Source: CAD feature listing. Evaluate the final solid. Frame: model axes, mm. A direction names the side the tool comes from. Coordinates: 2 decimals unless noted, no trailing zeros. Order: outer loops, then holes, each group sorted by start corner. A loop starts at its lowest first (then second) coordinate and runs counter-clockwise, first axis right, second up.
```python
from build123d import *

# Parameters (mm, degrees)
F0_R     = 1.5875
F0_W     = 8.89
F0_H     = 11.43
F0_W_2   = 11.43
F0_H_2   = 9.525
F1_DEPTH = 1.6
F0_H_3   = 1.905
F2_DEPTH = 10.9
F0_H_4   = 6.35
F3_DEPTH = 10.75


with BuildPart() as f1:
    # F0 (on Top) → F1 (new body)
    with BuildSketch(Plane.XY):
        Polygon((23.495, 0), (26.67, 0), (26.67, 66.04), (24.13, 66.04), (21.59, 68.58), (-11.176, 68.58), (-13.716, 66.04), (-25.146, 66.04), (-26.67, 64.516), (-26.67, 0), (-17.145, 0), (-17.145, 9.525), (-5.715, 9.525), (-5.715, 0), (14.605, 0), (14.605, 11.43), (23.495, 11.43), align=None)
        with Locations((-24.13, 15.24)):
            Circle(F0_R, mode=Mode.SUBTRACT)
        with Locations((24.13, 13.97)):
            Circle(F0_R, mode=Mode.SUBTRACT)
        with Locations((-8.89, 66.04)):
            Circle(F0_R, mode=Mode.SUBTRACT)
        with Locations((19.05, 66.04)):
            Circle(F0_R, mode=Mode.SUBTRACT)
        with Locations((19.05, 5.715)):
            Rectangle(F0_W, F0_H)
        with Locations((-11.43, 4.7625)):
            Rectangle(F0_W_2, F0_H_2)
    extrude(amount=-F1_DEPTH)

    # F0 (on Top) → F2 (join)
    with BuildSketch(Plane.XY):
        with Locations((19.05, 5.715)):
            Rectangle(F0_W, F0_H)
        with Locations((19.05, -0.9525)):
            Rectangle(F0_W, F0_H_3)
    extrude(amount=F2_DEPTH)

    # F0 (on Top) → F3 (join)
    with BuildSketch(Plane.XY):
        with Locations((-11.43, 4.7625)):
            Rectangle(F0_W_2, F0_H_2)
        with Locations((-11.43, -3.175)):
            Rectangle(F0_W_2, F0_H_4)
    extrude(amount=F3_DEPTH)


solid = f1.part
```
Q1. Set-up query: faces 4 (the flat face through (14.605, 5, 5)), 5 (the flat face through (-12, -3, 0)), 6 (the flat face through (-19, 66.04, -1)), 7 (the flat face through (19, -1.905, 5)), 8 (the flat face through (23.495, 5, 5)). Return all of +Z, -Z, +X, -X, +Y, -Y with unobstructed straight access to the full face (end or side cutting, diameter ignored); none if empty.
Solutions:
face 4: +Z, +Y, -Y
face 5: -Z, +X, -X, -Y
face 6: +Z, -Z, -X, +Y
face 7: +Z, -Z, +X, -Y
face 8: +Z, +X, +Y, -Y
Q2. Pull-direction query (Y, two-part tool) for faces 1 (the cylindrical face through (-9.097, 67.614, -0.789)), 2 (the flat face through (19, 5, 10.9)), 3 (the flat face through (19, 11.43, 5)); classes: pulls with the +Y half, pulls with the -Y half, needs draft (parallel to the pull), parting line crosses it, or undercut.
Solutions:
face 1: undercut
face 2: needs draft
face 3: pulls with the +Y half
Q3. Material intervals for line 1 along X through (y, z) = (1, 9) (3 decimals); line 2 along Y through (x, z) = (-24.13, -1); line 3 along Y through (x, z) = (-8.89, -0.9), sorted ascending.
Solutions:
line 1: x = -17.145 to -5.715, 14.605 to 23.495
line 2: y = 0 to 13.65, 16.83 to 66.04
line 3: y = 0 to 64.45, 67.63 to 68.58
Q4. Section query A-A on x = -24.13. Output: boundary loops of the cut face in (y, z).
Solutions:
outline: (0, -1.6) - (13.65, -1.6) - (13.65, 0) - (0, 0) - close; (16.83, -1.6) - (66.04, -1.6) - (66.04, 0) - (16.83, 0) - close
Q5. Pin query (flat end, axial travel): P1, Ø1.9, axis at x = 24.13, y = 13.97, coming from the -Z side; P2, Ø2.5, axis at x = 18.5, z = 6, coming from the +Y side; P3, Ø0.5, axis at x = -13, z = -1, coming from the -Y side; P4, Ø4, axis at y = 2, z = 8.5, coming from the -X side (3 decimals). Return the tip coordinate at first contact, or that it passes through.
Solutions:
P1: passes through
P2: stops at y = 11.43
P3: stops at y = 0
P4: stops at x = -17.145
Q6. Section query C-C on y = 7.5. Output: boundary loops of the cut face in (x, z) (3 decimals).
Solutions:
outline: (-26.67, -1.6) - (26.67, -1.6) - (26.67, 0) - (23.495, 0) - (23.495, 10.9) - (14.605, 10.9) - (14.605, 0) - (-5.715, 0) - (-5.715, 10.75) - (-17.145, 10.75) - (-17.145, 0) - (-26.67, 0) - close
Q7. Section query B-B on z = 6. Output: boundary loops of the cut face in (x, y) (3 decimals), plus the area to 3 significant figures.
Solutions:
outline: (-17.145, -6.35) - (-5.715, -6.35) - (-5.715, 9.525) - (-17.145, 9.525) - close; (14.605, -1.905) - (23.495, -1.905) - (23.495, 11.43) - (14.605, 11.43) - close
area: 300 mm2
